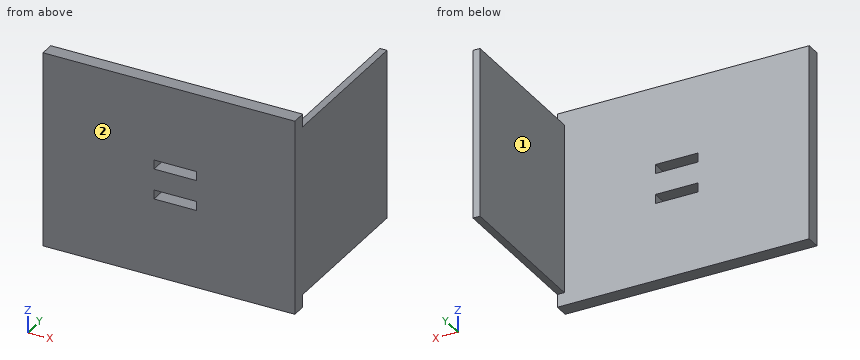
Autodesk Inventor part; units mm, degrees
ref_plane "YZ Plane" through (0, 0, 0) normal (1, 0, 0) x (0, 1, 0)
ref_plane "XZ Plane" through (0, 0, 0) normal (0, 1, 0) x (-1, 0, 0)
ref_plane "XY Plane" through (0, 0, 0) normal (0, 0, 1) x (1, 0, 0)
sketch "Sketch1" plane through (0, 0, 0) normal (0, 1, 0) x (-1, 0, 0)
  line L0 (53.2003, -37.719) -> (-53.2003, -37.719)
  line L1 (-53.2003, -37.719) -> (-53.2003, 37.719)
  line L2 (-53.2003, 37.719) -> (53.2003, 37.719)
  line L3 (53.2003, 37.719) -> (53.2003, -37.719)
  line L4 (53.2003, -37.719) -> (-53.2003, 37.719) construction
  line L5 (-53.2003, -37.719) -> (53.2003, 37.719) construction
  point P0 (0, 0)
  dimension "d0" = 106.4006
  dimension "d1" = 75.438
extrude "Extrusion1" add sketch "Sketch1" along normal blind 6.35
sketch "Sketch2" plane through (0, 6.35, 0) normal (0, 1, 0) x (1, 0, 0)
  line L0 (53.2003, -37.719) -> (53.2003, 37.719)
  line L1 (53.2003, -37.719) -> (53.2003, -34.544)
  line L2 (53.2003, -34.544) -> (50.0761, -34.544)
  line L3 (53.2003, 37.719) -> (53.2003, 34.544)
  line L4 (53.2003, 34.544) -> (50.0761, 34.544)
  line L5 (50.0761, 34.544) -> (50.0761, -34.544)
  line L6 (53.2003, -34.544) -> (53.2003, 34.544)
  point P0 (0, 0)
  dimension "d4" = 3.175
  dimension "d5" = 3.1242
  dimension "d6" = 3.175
extrude "Extrusion2" add sketch "Sketch2" along normal blind 68.58
fillet "Fillet1" radius 3.175 1 edges at (50.0761, 6.35, 0)
sketch "Sketch3" plane through (0, 0, 0) normal (0, -1, 0) x (1, 0, 0)
  line L0 (-9.525, 8.763) -> (9.525, 8.763)
  line L1 (9.525, 8.763) -> (9.525, -8.763)
  line L2 (9.525, -8.763) -> (-9.525, -8.763)
  line L3 (-9.525, -8.763) -> (-9.525, 8.763)
  line L4 (-9.525, 8.763) -> (9.525, -8.763) construction
  line L5 (9.525, 8.763) -> (-9.525, -8.763) construction
  line L6 (9.525, -8.763) -> (-9.525, -8.763)
  line L7 (-9.525, -8.763) -> (-9.525, -4.699)
  line L8 (-9.525, -4.699) -> (9.525, -4.699)
  line L9 (9.525, -4.699) -> (9.525, -8.763)
  line L10 (9.525, 8.763) -> (-9.525, 8.763)
  line L11 (-9.525, 8.763) -> (-9.525, 4.699)
  line L12 (-9.525, 4.699) -> (9.525, 4.699)
  line L13 (9.525, 4.699) -> (9.525, 8.763)
  point P0 (0, 0)
  dimension "d10" = 19.05
  dimension "d11" = 17.526
  dimension "d12" = 4.064
  dimension "d13" = 4.064
extrude "Extrusion3" cut sketch "Sketch3" against normal blind 68.58 contours L0 L1 L12 L3 | L8 L1 L2 L3
sketch "Sketch4" plane through (0, 0, 0) normal (0, -1, 0) x (1, 0, 0)
  point P0 (0, 0)
sketch "Sketch5" plane through (0, 0, 0) normal (0, -1, 0) x (1, 0, 0)
  point P0 (0, 0)
sketch "Sketch6" plane through (53.2003, 0, -37.719) normal (0, 0, -1) x (-1, 0, 0)
  line L0 (106.4006, 0) -> (0, 0)
  line L1 (0, 6.35) -> (106.4006, 6.35)
  line L2 (106.4006, 0) -> (0, 0)
  line L3 (0, 0) -> (0, 6.35)
  line L4 (0, 6.35) -> (106.4006, 6.35)
  line L5 (106.4006, 6.35) -> (106.4006, 0)
  point P0 (53.2003, 0)
sketch "Sketch7" plane through (0, 6.35, 0) normal (0, 1, 0) x (1, 0, 0)
  line L0 (53.2003, 34.544) -> (53.2003, 37.719)
  line L1 (46.9519, -37.719) -> (53.2003, -37.719)
  line L2 (53.2003, -37.719) -> (53.2003, 37.719)
  line L3 (53.2003, 37.719) -> (46.9519, 37.719)
  line L4 (46.9519, 37.719) -> (46.9519, -37.719)
  line L5 (50.0761, 34.544) -> (50.0761, -34.544)
  line L6 (46.9519, -37.719) -> (53.2003, 37.719) construction
  line L7 (53.2003, -37.719) -> (46.9519, 37.719) construction
  point P0 (0, 0)
  point P1 (50.0761, 0)
extrude "Extrusion4" add sketch "Sketch7" along normal blind 68.58
sketch "Sketch8" plane through (0, 74.93, 0) normal (0, 1, 0) x (1, 0, 0)
  line L0 (53.2003, -37.719) -> (53.2003, 37.719)
  line L1 (53.2003, 37.719) -> (46.9519, 37.719)
  line L2 (53.2003, -37.719) -> (50.0761, -37.719)
  line L3 (50.0761, -37.719) -> (50.0761, 37.719)
  line L4 (50.0761, 37.719) -> (53.2003, 37.719)
  line L5 (53.2003, 37.719) -> (53.2003, -37.719)
  line L6 (46.9519, -37.719) -> (53.2003, -37.719)
  line L7 (50.0761, 37.719) -> (46.9519, 37.719)
  line L8 (46.9519, 37.719) -> (46.9519, -37.719)
  line L9 (46.9519, -37.719) -> (50.0761, -37.719)
  line L10 (50.0761, -37.719) -> (50.0761, 37.719)
  point P0 (0, 0)
extrude "Extrusion5" cut sketch "Sketch8" against normal blind 68.58 contours L6 L8 L1 L3
sketch "Sketch9" plane through (53.2003, 0, -37.719) normal (0, 0, -1) x (-1, 0, 0)
  line L0 (3.1242, 6.35) -> (106.4006, 6.35)
  line L1 (106.4006, 6.35) -> (0, 6.35)
  line L2 (0, 6.35) -> (0, 0)
  line L3 (0, 0) -> (106.4006, 0)
  line L4 (106.4006, 0) -> (106.4006, 6.35)
  point P0 (53.2003, 0)
extrude "Extrusion6" add sketch "Sketch9" along normal blind 5.715
sketch "Sketch10" plane through (-53.2003, 0, 37.719) normal (0, 0, 1) x (1, 0, 0)
  line L0 (0, 6.35) -> (106.4006, 6.35)
  line L1 (106.4006, 0) -> (106.4006, 74.93)
  line L2 (0, 6.35) -> (106.4006, 6.35)
  line L3 (106.4006, 6.35) -> (106.4006, 0)
  line L4 (106.4006, 0) -> (0, 0)
  line L5 (0, 0) -> (0, 6.35)
  point P0 (53.2003, 0)
extrude "Extrusion7" add sketch "Sketch10" along normal blind 5.715
sketch "Sketch11" plane through (-53.2003, 0, -43.434) normal (-1, 0, 0) x (0, 0, 1)
  line L0 (0, 0) -> (0, 6.35)
  line L1 (86.868, 0) -> (0, 0)
  line L2 (0, 6.35) -> (86.868, 6.35)
  line L3 (86.868, 6.35) -> (86.868, 0)
  line L4 (86.868, 0) -> (0, 0)
  line L5 (0, 0) -> (0, 6.35)
  point P0 (43.434, 0)
extrude "Extrusion8" add sketch "Sketch11" along normal blind 5.715
properties part number "Boxpt2"
Design review of the part built by this model. Coordinates are the model's own, in mm. Face numbers are marked on the shaded views. A direction names the side the tool comes from. Coordinates: 2 decimals unless noted, no trailing zeros. Loops run counter-clockwise (first coordinate to the right, second up) from the corner with the lowest first, then second, coordinate; pieces in that order, holes last.
Q1. Tool access review of the marked faces 1 and 2: name each direction out of +Z, -Z, +X, -X, +Y, -Y from which nothing blocks a thin tool from reaching the whole face with its end or side.
Reported:
face 1: +Z, -Z, -X, +Y
face 2: +Z, -Z, +X, -X, -Y
Q2. We need section C-C on y = 43.5. State the section outline as (x, z) points.
Reported:
outline: (50.08, -37.72) - (53.2, -37.72) - (53.2, 37.72) - (50.08, 37.72) - close
Q3. We need section D-D on x = 13.5. State the section outline as (y, z) points.
Reported:
outline: (0, -43.43) - (6.35, -43.43) - (6.35, 43.43) - (0, 43.43) - close
Q4. To check wall thickness, follow line 1 (X direction, y = 14.5, z = -17); line 2 (Y direction, x = -10, z = 35.5). State the ranges of each line that lie inside material, in increasing order.
Reported:
line 1: x = 50.08 to 53.2
line 2: y = 0 to 6.35
Q5. We need section A-A on x = -7. State the section outline as (y, z) points, and give its area (3 significant figures).
Reported:
outline: (0, -43.43) - (6.35, -43.43) - (6.35, -8.76) - (0, -8.76) - close; (0, -4.7) - (6.35, -4.7) - (6.35, 4.7) - (0, 4.7) - close; (0, 8.76) - (6.35, 8.76) - (6.35, 43.43) - (0, 43.43) - close
area: 500 mm2
Q6. For pin 1 (2.5 mm diameter, centred on x = 51.5, y = 47.5, fed in from +Z); pin 2 (0.9 mm diameter, centred on x = 51, y = 34.5, fed in from -Z); pin 3 (4 mm diameter, centred on x = 12, z = 3.5, fed in from +Y), all flat-tipped, find the tip position at first contact; note any pin that passes through.
Reported:
pin 1: stops at z = 37.72
pin 2: stops at z = -37.72
pin 3: stops at y = 6.35
